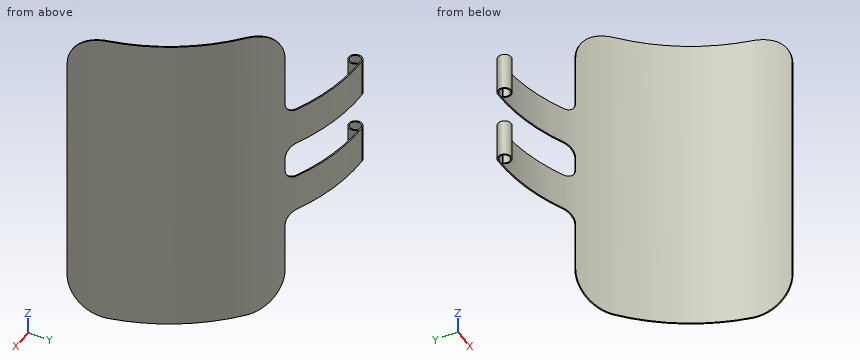
```python
from build123d import *

# Parameters (mm, degrees)
BOSS_EXTRUDE1_DEPTH = 125
CUT_EXTRUDE1_DEPTH  = 15
CUT_EXTRUDE2_DEPTH  = 80
FILLET1_START       = 83.934299194
FILLET1_DEPTH       = 68.065700806
FILLET1_START_2     = 78.711006452
FILLET1_2_DEPTH     = 73.288993548
FILLET2_R           = 10


with BuildPart() as part:
    # Sketch2 → Boss-Extrude1 (new, symmetric)
    with BuildSketch(Plane.XY):
        with BuildLine():
            Line((3.00520382, 148.75520382), (3.712310601, 149.462310601))
            ThreePointArc((3.712310601, 149.462310601), (-2.00908802, 140.899632454), (0, 151))
            ThreePointArc((0, 151), (106.773123959, 106.773123959), (151, 0))
            Line((151, 0), (150, 0))
            ThreePointArc((150, 0), (106.066017178, 106.066017178), (0, 150))
            ThreePointArc((0, 150), (-1.626404588, 141.823511987), (3.00520382, 148.75520382))
        make_face()
    extrude(amount=BOSS_EXTRUDE1_DEPTH, both=True)

    # Sketch3 → Cut-Extrude1 (cut, symmetric)
    with BuildSketch(Plane.XY):
        with BuildLine():
            Line((75, 129.903810568), (75.5, 130.769835971))
            ThreePointArc((75.5, 130.769835971), (39.08167581, 145.85479977), (0, 151))
            ThreePointArc((0, 151), (-2.00908802, 140.899632454), (3.712310601, 149.462310601))
            Line((3.712310601, 149.462310601), (3.00520382, 148.75520382))
            ThreePointArc((3.00520382, 148.75520382), (-1.626404588, 141.823511987), (0, 150))
            ThreePointArc((0, 150), (38.822856765, 144.888873943), (75, 129.903810568))
        make_face()
    extrude(amount=CUT_EXTRUDE1_DEPTH, both=True, mode=Mode.SUBTRACT)

    # Sketch4 → Cut-Extrude2 (cut)
    with BuildSketch(Plane.XY.offset(125)):
        with BuildLine():
            Line((75, 129.903810568), (75.5, 130.769835971))
            ThreePointArc((75.5, 130.769835971), (39.08167581, 145.85479977), (0, 151))
            ThreePointArc((0, 151), (-2.00908802, 140.899632454), (3.712310601, 149.462310601))
            Line((3.712310601, 149.462310601), (3.00520382, 148.75520382))
            ThreePointArc((3.00520382, 148.75520382), (-1.626404588, 141.823511987), (0, 150))
            ThreePointArc((0, 150), (38.822856765, 144.888873943), (75, 129.903810568))
        make_face()
    cut_extrude2 = extrude(amount=-CUT_EXTRUDE2_DEPTH, mode=Mode.SUBTRACT)

    # Mirror1: Cut-Extrude2 across plane
    add(cut_extrude2.mirror(Plane.XY), mode=Mode.SUBTRACT)

    # Fillet1: read off the stored shape, not the designer's step
    # Fillet1 outline → Fillet1 (cut)
    with BuildSketch(Plane(origin=(0, 0, 0), x_dir=(0.8660254037844386, -0.4999999999999999, 0), z_dir=(0.4999999999999999, 0.8660254037844388, 0)).offset(FILLET1_START)):
        with BuildLine():
            Line((0, 125), (0, 95))
            ThreePointArc((0, 95), (8.786796564, 116.213203436), (30, 125))
            Line((30, 125), (0, 125))
        make_face()
        with BuildLine():
            Line((0, -125), (30, -125))
            ThreePointArc((30, -125), (8.786796564, -116.213203436), (0, -95))
            Line((0, -95), (0, -125))
        make_face()
    extrude(amount=FILLET1_DEPTH, mode=Mode.SUBTRACT)

    # Fillet1 2 outline → Fillet1 2 (cut)
    with BuildSketch(Plane.YZ.offset(FILLET1_START_2)):
        with BuildLine():
            ThreePointArc((30, -125), (8.786796564, -116.213203436), (0, -95))
            Line((0, -95), (0, -125))
            Line((0, -125), (30, -125))
        make_face()
        with BuildLine():
            Line((0, 125), (0, 95))
            ThreePointArc((0, 95), (8.786796564, 116.213203436), (30, 125))
            Line((30, 125), (0, 125))
        make_face()
    extrude(amount=FILLET1_2_DEPTH, mode=Mode.SUBTRACT)

    # Fillet2
    fillet2_edges = [part.edges().sort_by_distance(p)[0] for p in [
        (75.25, 130.33682327, -15),
        (75.25, 130.33682327, 15),
        (75.25, 130.33682327, 45),
        (75.25, 130.33682327, -45),
    ]]
    fillet(fillet2_edges, radius=FILLET2_R)


solid = part.part
```
For this review, take the finished solid that the model builds, in its own axes (mm). Give positions to 0.01 mm unless a question says otherwise; leave off trailing zeros. Order: outer loops, then holes, each group sorted by start corner. A loop starts at its lowest first (then second) coordinate and runs counter-clockwise, first axis right, second up.
1) Insertion check: pin 1 (8 mm diameter, centred on x = 90.5, z = 33.5, fed in from -Y); pin 2 (6 mm diameter, centred on y = 44, z = 49, fed in from -X); pin 3 (18 mm diameter, centred on x = 34.5, y = 146, fed in from +Z); pin 4 (7.5 mm diameter, centred on x = 0, y = 145.75, fed in from -Z). Each pin has a flat end and moves straight along its axis. Give the tip position at first contact, or say it passes through.
2) Take a section at C-C (z = -41). Give the boundary of the cut face in (x, y), then the cut area to 3 significant figures.
3) Take a section at B-B (y = 145.75). Give the boundary of the cut face in (x, z).
4) Take a section at D-D (y = 87). Give the boundary of the cut face in (x, z).
5) Wall thickness on line 1 (Y direction, x = 0, z = -33); line 2 (X direction, y = 69, z = -95); line 3 (X direction, y = 75.5, z = -105): over which ranges is each line inside the solid? List them lowest first.
6) Take a section at A-A (x = 19). Give the boundary of the cut face in (y, z), then the cut area to 3 significant figures.
Derived:
1. pin 1: stops at y = 116.49
1. pin 2: stops at x = 142.45
1. pin 3: stops at z = 45
1. pin 4: passes through
2. outline: (0, 150) arc R150 cw to (150, 0) - (151, 0) arc R151 ccw to (0, 151) arc R5.25 ccw (long way) to (3.71, 149.46) - (3.01, 148.76) arc R4.25 cw (long way) to start
2. area: 263 mm2
3. outline: (-5.25, -45) - (-4.25, -45) - (-4.25, -15) - (-5.25, -15) - close; (-5.25, 15) - (-4.25, 15) - (-4.25, 45) - (-5.25, 45) - close; (4.25, -45) - (5.25, -45) - (5.25, -15) - (4.25, -15) - close; (4.25, 15) - (5.25, 15) - (5.25, 45) - (4.25, 45) - close; (35.45, -45) - (39.47, -45) - (39.47, -15) - (35.45, -15) - close; (35.45, 15) - (39.47, 15) - (39.47, 45) - (35.45, 45) - close
4. outline: (122.19, -125) - (123.42, -125) - (123.42, 125) - (122.19, 125) - close
5. line 1: y = 140.5 to 141.5, 150 to 151
5. line 2: x = 133.19 to 134.31
5. line 3: x = 129.61 to 130.77
6. outline: (148.79, -45) - (149.8, -45) - (149.8, -15) - (148.79, -15) - close; (148.79, 15) - (149.8, 15) - (149.8, 45) - (148.79, 45) - close
6. area: 60.5 mm2
